Autodesk Inventor part; units mm, degrees
ref_plane "YZ Plane" through (0, 0, 0) normal (1, 0, 0) x (0, 1, 0)
ref_plane "XZ Plane" through (0, 0, 0) normal (0, 1, 0) x (-1, 0, 0)
ref_plane "XY Plane" through (0, 0, 0) normal (0, 0, 1) x (1, 0, 0)
sketch "Sketch1" plane through (0, 0, 0) normal (0, 0, 1) x (1, 0, 0)
  arc A0 (5, 0) -> (0, 5) centre (0, 0) ccw
  arc A1 (6.5, 0) -> (0, 6.5) centre (0, 0) ccw
  line L0 (7, -6.5) -> (15, -6.5)
  line L1 (7.5, -5) -> (15, -5)
  line L2 (15, -5) -> (15, -6.5)
  line L3 (6.5, 0) -> (6.5, -4)
  line L4 (0, 10.9318) -> (0, -12.0627) construction
  line L5 (5, 0) -> (5, -4.5)
  arc A2 (5, -4.5) -> (7, -6.5) centre (7, -4.5) ccw
  arc A3 (6.5, -4) -> (7.5, -5) centre (7.5, -4) ccw
  arc A4 (0, 5) -> (-5, 0) centre (0, 0) ccw
  arc A5 (0, 6.5) -> (-6.5, 0) centre (0, 0) ccw
  line L6 (-7, -6.5) -> (-15, -6.5)
  line L7 (-7.5, -5) -> (-15, -5)
  line L8 (-15, -5) -> (-15, -6.5)
  line L9 (-6.5, 0) -> (-6.5, -4)
  line L10 (-5, 0) -> (-5, -4.5)
  arc A6 (-7, -6.5) -> (-5, -4.5) centre (-7, -4.5) ccw
  arc A7 (-7.5, -5) -> (-6.5, -4) centre (-7.5, -4) ccw
  dimension "d0" = 10
  dimension "d1" = 1.5
  dimension "d4" = 2
  dimension "d5" = 1
extrude "Extrusion1" add sketch "Sketch1" along normal mid plane 50
sketch "Sketch2" plane through (7.5, -5, 25) normal (0, 1, 0) x (1, 0, 0)
  circle A0 centre (-18.75, 3.75) radius 1.5
  circle A1 centre (3.75, 3.75) radius 1.5
  line L0 (7.5, 50) -> (7.5, 0)
  line L1 (-26.7627, 25) -> (16.6618, 25) construction
  circle A2 centre (-18.75, 46.25) radius 1.5
  circle A3 centre (3.75, 46.25) radius 1.5
  point P0 (-7.5, 25)
extrude "Extrusion2" cut sketch "Sketch2" against normal up to next
sketch "Sketch3" plane through (0, 0, 0) normal (1, 0, 0) x (0, 1, 0)
  line L0 (-5, 25) -> (-5, -25) construction
  line L1 (-5, -13) -> (11.6912, -13)
  line L2 (11.6912, -13) -> (11.6912, -8)
  line L3 (11.6912, -8) -> (-5, -8)
  line L4 (-5, 4) -> (11.6912, 4)
  line L5 (11.6912, 4) -> (11.6912, 9)
  line L6 (11.6912, 9) -> (-5, 9)
  line L7 (-5, 4) -> (-5, 9)
  line L8 (-5, -13) -> (-5, -8)
  point P0 (0, 0)
  dimension "d16" = 5
  dimension "d17" = 12
  dimension "d18" = 5
  dimension "d19" = 12
extrude "Extrusion3" cut sketch "Sketch3" along normal mid plane 50
sketch "Sketch4" plane through (0, 0, 0) normal (0, 1, 0) x (-1, 0, 0)
  line L0 (2.5, 6.6372) -> (-2.5, 6.6372)
  line L1 (-2.5, 6.6372) -> (-2.5, -10.1613)
  line L2 (-2.5, -10.1613) -> (2.5, -10.1613)
  line L3 (2.5, -10.1613) -> (2.5, 6.6372)
  line L4 (2.5, 6.6372) -> (-2.5, -10.1613) construction
  line L5 (-2.5, 6.6372) -> (2.5, -10.1613) construction
  point P0 (0, 0)
  point P1 (0, -1.7621)
  dimension "d22" = 5
extrude "Extrusion4" cut sketch "Sketch4" along normal up to next
The listing builds one solid part. Answer for the finished solid, in the listing's coordinates (mm). A direction names the side the tool comes from. Give positions to 0.01 mm unless a question says otherwise; leave off trailing zeros. Loops run counter-clockwise (first coordinate to the right, second up) from the corner with the lowest first, then second, coordinate; pieces in that order, holes last. Notation, with made-up numbers: M -13.5,87.25 L 12.5,87.25 A22 cw 12.5,106.25 Z; hole C 63.5,42.25 d10. An arc over 180 degrees is marked long. One line per item, written item: value.
1. For faces 1 (the face through (-2, 5, 9)), 2 (the face through (5, -2, 17)), 3 (the face through (-6.5, -2, -19)), determine the directions among +Z, -Z, +X, -X, +Y, -Y from which every point of the face is accessible in a straight line to the end or side of a thin tool.
Found:
face 1: +X, -X, +Y
face 2: +Z, -Z, -Y
face 3: +Z, -Z, -X, +Y
2. Section C-C on z = -10.5 is taken. Determine the outline of the cut face in (x, y).
Found:
outline: M -15,-6.5 L -7,-6.5 A2 ccw -5.06,-5 L -15,-5 Z; M 5.06,-5 A2 ccw 7,-6.5 L 15,-6.5 L 15,-5 Z
3. Find the intervals of material crossed by probe 1 along Z at (x, y) = (-11.25, -5.4); probe 2 along Z at (x, y) = (5.5, 0.75); probe 3 along X at (y, z) = (-3, 9.5), in increasing order.
Found:
probe 1: -25 to -22.75, -19.75 to 19.75, 22.75 to 25
probe 2: -25 to -13, -8 to 4, 9 to 25
probe 3: -6.5 to -5, 5 to 6.5
4. Section D-D on x = 0 is taken. Determine the outline of the cut face in (y, z), plus the area to 3 significant figures.
Found:
outline: M 5,-25 L 6.5,-25 L 6.5,-13 L 5,-13 Z; M 5,9 L 6.5,9 L 6.5,25 L 5,25 Z
area: 42.0 mm^2
5. Each of these flat-tipped pins is pushed along its axis until it touches: P1, Ø1.3, axis at y = -2.5, z = -19, coming from the -X side; P2, Ø2.5, axis at y = -1.5, z = 14.5, coming from the +X side; P3, Ø4.5, axis at y = -2.5, z = 14.5, coming from the +X side. Where does it stop, or does it pass through?
Found:
P1: x = -6.5
P2: x = 6.5
P3: x = 6.84
6. Section A-A on z = -21.25 is taken. Determine the outline of the cut face in (x, y), plus the area to 3 significant figures.
Found:
outline: M -15,-6.5 L -12.75,-6.5 L -12.75,-5 L -15,-5 Z; M -9.75,-6.5 L -7,-6.5 A2 ccw -5,-4.5 L -5,0 A5 cw 5,0 L 5,-4.5 A2 ccw 7,-6.5 L 9.75,-6.5 L 9.75,-5 L 7.5,-5 A1 cw 6.5,-4 L 6.5,0 A6.5 ccw -6.5,0 L -6.5,-4 A1 cw -7.5,-5 L -9.75,-5 Z; M 12.75,-6.5 L 15,-6.5 L 15,-5 L 12.75,-5 Z
area: 61.8 mm^2
7. Section B-B on y = -3 is taken. Determine the outline of the cut face in (x, z).
Found:
outline: M -6.5,-25 L -5,-25 L -5,-13 L -6.5,-13 Z; M -6.5,-8 L -5,-8 L -5,4 L -6.5,4 Z; M -6.5,9 L -5,9 L -5,25 L -6.5,25 Z; M 5,-25 L 6.5,-25 L 6.5,-13 L 5,-13 Z; M 5,-8 L 6.5,-8 L 6.5,4 L 5,4 Z; M 5,9 L 6.5,9 L 6.5,25 L 5,25 Z
